from build123d import *

# Parameters (mm, degrees)
SKETCH_1_R          = 12
EXTRUDE_1_DEPTH     = 6
SKETCH_2_R          = 12
EXTRUDE_2_DEPTH     = 3.6
SKETCH_3_R          = 3
CUT_EXTRUDE_1_DEPTH = 20.497692171
CUT_EXTRUDE_2_DEPTH = 6
CHAMFER_1_SIZE      = 0.5
SKETCH_5_R          = 1.25
CUT_EXTRUDE_3_DEPTH = 23.184679398
CUT_EXTRUDE_7_DEPTH = 0.5
SKETCH_13_R         = 1.25
CUT_EXTRUDE_8_DEPTH = 23.184679398
SKETCH_8_R          = 1.25
CUT_EXTRUDE_9_DEPTH = 20.49769222


with BuildPart() as part:
    # 草图1 → 凸台-拉伸1 (new body)
    with BuildSketch(Plane(origin=(0, 0, 0), x_dir=(0, 0, -1), z_dir=(1, 0, 0))):
        Circle(SKETCH_1_R)
    extrude(amount=EXTRUDE_1_DEPTH)

    # 草图2 → 凸台-拉伸2 (add)
    with BuildSketch(Plane(origin=(6, 0, 0), x_dir=(0, 0, -1), z_dir=(1, 0, 0))):
        Circle(SKETCH_2_R)
    extrude(amount=EXTRUDE_2_DEPTH)

    # 草图3 → 切除-拉伸1 (cut, through all)
    with BuildSketch(Plane.ZY):
        Circle(SKETCH_3_R)
    extrude(amount=-CUT_EXTRUDE_1_DEPTH, mode=Mode.SUBTRACT)

    # 草图4 → 切除-拉伸2 (cut)
    with BuildSketch(Plane.ZY):
        with BuildLine():
            Line((-11.832159566, 2), (11.832159566, 2))
            ThreePointArc((11.832159566, 2), (0, 12), (-11.832159566, 2))
        make_face()
        with BuildLine():
            Line((11.313708499, -4), (-11.313708499, -4))
            ThreePointArc((-11.313708499, -4), (0, -12), (11.313708499, -4))
        make_face()
    extrude(amount=-CUT_EXTRUDE_2_DEPTH, mode=Mode.SUBTRACT)

    # 倒角1
    chamfer_1_edges = [part.edges().sort_by_distance(p)[0] for p in [
        (0, -1.033052698, 11.955450729),
        (0, -2.029223745, -11.827182716),
    ]]
    chamfer(chamfer_1_edges, length=CHAMFER_1_SIZE)

    # 草图5 → 切除-拉伸3 (cut, through all)
    with BuildSketch(Plane.XZ.offset(4)):
        with Locations(Location((3, -7, 0), (0, 0, 270))):
            Circle(SKETCH_5_R)
        with Locations(Location((3, 7, 0), (0, 0, 270))):
            Circle(SKETCH_5_R)
    extrude(amount=-CUT_EXTRUDE_3_DEPTH, mode=Mode.SUBTRACT)

    # 草图12 → 切除-拉伸7 (cut)
    with BuildSketch(Plane.ZY.offset(-6)):
        with BuildLine():
            Line((11.313708499, -4), (-11.313708499, -4))
            ThreePointArc((-11.313708499, -4), (0, -12), (11.313708499, -4))
        make_face()
        with BuildLine():
            Line((2.236067977, 2), (11.832159566, 2))
            ThreePointArc((11.832159566, 2), (0, 12), (-11.832159566, 2))
            Line((-11.832159566, 2), (-2.236067977, 2))
            ThreePointArc((-2.236067977, 2), (0, 3), (2.236067977, 2))
        make_face()
    extrude(amount=-CUT_EXTRUDE_7_DEPTH, mode=Mode.SUBTRACT)

    # 草图13 → 切除-拉伸8 (cut, through all)
    with BuildSketch(Plane(origin=(0, -4, 0), x_dir=(-1, 0, 0), z_dir=(0, -1, 0))):
        with Locations(Location((-2.6, 0, 0), (0, 0, 90))):
            Circle(SKETCH_13_R)
    extrude(amount=-CUT_EXTRUDE_8_DEPTH, mode=Mode.SUBTRACT)

    # 草图8 → 切除-拉伸9 (cut, through all)
    with BuildSketch(Plane(origin=(9.6, 0, 0), x_dir=(0, 0, -1), z_dir=(1, 0, 0))):
        with Locations((0, 9)):
            Circle(SKETCH_8_R)
        with Locations((0, -9)):
            Circle(SKETCH_8_R)
    extrude(amount=-CUT_EXTRUDE_9_DEPTH, mode=Mode.SUBTRACT)


solid = part.part
Build history of the part. All positions in model axes, mm. A direction names the side the tool comes from. Round coordinates to 2 decimals unless told otherwise and drop trailing zeros. Write each loop counter-clockwise with the first axis right and the second up, starting at its lowest first coordinate (ties: lowest second). Pieces come first, ordered by that corner, then holes. Notation, with made-up numbers: (81.5, 57) -> (140.5, 57) arc R21 ccw to (140.5, 71) -> close; hole circle Ø1 at (66, 78.25). An arc over 180 degrees is marked (long way). Use one line per item in the form item = value.
Q1. Tool access for faces 1 (the flat face through (5, -4, 0)), 2 (the flat face through (6.5, 6, 0)), 3 (the flat face through (9.6, -2.5, -2.5)): list every direction of +Z, -Z, +X, -X, +Y, -Y with a clear straight run to the whole face (end or side of a thin tool).
Conclusion:
face_1 = +Z, -Z, -X, -Y
face_2 = +Z, -Z, -X, +Y
face_3 = +Z, -Z, +X, +Y, -Y
Q2. Drop flat-ended pins along their axis: P1, Ø3, axis at x = 8, z = 8.5, coming from the +Y side; P2, Ø3, axis at x = 2.5, z = 8, coming from the +Y side; P3, Ø1.5, axis at x = 5.5, y = 1.5, coming from the +Z side. Give the stop position or say it passes through.
Conclusion:
P1 = 9.75
P2 = 2
P3 = 11.98
Q3. Band-saw the part on B-B, the plane z = 7. Write the cut outline in (x, y).
Conclusion:
outline = (0, -4) -> (1.75, -4) -> (1.75, 2) -> (0, 2) -> close; (4.25, -4) -> (6.5, -4) -> (6.5, -9.75) -> (9.6, -9.75) -> (9.6, 9.75) -> (6.5, 9.75) -> (6.5, 2) -> (4.25, 2) -> close
Q4. Drill centre lines: L1, parallel to Y at x = 7.8, z = 0; L2, parallel to X at y = 0.8, z = 7; L3, parallel to X at y = -3.1, z = 0. Where is each one in solid material? Low to high.
Conclusion:
L1 = -12 to -10.25, -7.75 to -3, 3 to 7.75, 10.25 to 12
L2 = 0 to 1.75, 4.25 to 9.6
L3 = 0 to 1.35, 3.85 to 9.6
Q5. Band-saw the part on A-A, the plane y = 0. Write the cut outline in (x, z), then the cut area to 3 significant figures.
Conclusion:
outline = (0, -11.5) -> (0.5, -12) -> (9.6, -12) -> (9.6, -3) -> (0, -3) -> close; (0, 3) -> (9.6, 3) -> (9.6, 12) -> (0.5, 12) -> (0, 11.5) -> close; hole circle Ø2.5 at (3, -7); hole circle Ø2.5 at (3, 7)
area = 163 mm²
Q6. Band-saw the part on D-D, the plane y = 8.5. Write the cut outline in (x, z), then the cut area to 3 significant figures.
Conclusion:
outline = (6.5, -8.47) -> (9.6, -8.47) -> (9.6, -1.15) -> (6.5, -1.15) -> close; (6.5, 1.15) -> (9.6, 1.15) -> (9.6, 8.47) -> (6.5, 8.47) -> close
area = 45.4 mm²
Q7. Band-saw the part on C-C, the plane x = 2.6. Write the cut outline in (y, z).
Conclusion:
outline = (-4, -11.31) arc R12 ccw to (2, -11.83) -> (2, -8.18) -> (-4, -8.18) -> close; (-4, -5.82) -> (2, -5.82) -> (2, -2.24) arc R3 cw to (-2.73, -1.25) -> (-4, -1.25) -> close; (-4, 1.25) -> (-2.73, 1.25) arc R3 cw to (2, 2.24) -> (2, 5.82) -> (-4, 5.82) -> close; (-4, 8.18) -> (2, 8.18) -> (2, 11.83) arc R12 ccw to (-4, 11.31) -> close
Q8. Two-plate mould, pull along Y, no slides. Class faces 4 (the cylindrical face through (5.799, -2.662, 1.384)), 5 (the flat face through (4, 2, -8)), 6 (the conical face through (0.19, -1.1, -11.64)): released by +Y, released by -Y, zero draft, split by the parting line, or undercut.
Conclusion:
face_4 = undercut
face_5 = released by +Y
face_6 = split by the parting line
